Can you work these out from the model? Positions are in its coordinate system, mm. A direction names the side the tool comes from. Coordinates: 2 decimals unless noted, no trailing zeros. Write each loop counter-clockwise with the first axis right and the second up, starting at its lowest first coordinate (ties: lowest second). Pieces come first, ordered by that corner, then holes. Notation, with made-up numbers: (-6, -16) -> (1, -16) arc R15 ccw to (1, 10) -> close; hole circle Ø8 at (47.25, 84.5). An arc over 180 degrees is marked (long way). Use one line per item in the form item = value.
```python
from build123d import *

# Parameters (mm, degrees)
SKETCH1_W           = 110.236
SKETCH1_H           = 89.916
BOSS_EXTRUDE1_DEPTH = 17.78
SKETCH2_W           = 19.05
SKETCH2_H           = 12.7
CUT_EXTRUDE1_DEPTH  = 17.78


with BuildPart() as part:
    # Sketch1 → Boss-Extrude1 (new body)
    with BuildSketch(Plane(origin=(0, 0, 0), x_dir=(1, 0, 0), z_dir=(0, 1, 0))):
        with Locations((0, -19.671907216)):
            Rectangle(SKETCH1_W, SKETCH1_H)
    extrude(amount=BOSS_EXTRUDE1_DEPTH)

    # Sketch2 → Cut-Extrude1 (cut)
    with BuildSketch(Plane(origin=(0, 17.78, 0), x_dir=(1, 0, 0), z_dir=(0, 1, 0))):
        with Locations((-45.593, -58.279907216)):
            Rectangle(SKETCH2_W, SKETCH2_H)
        with Locations((45.593, -58.279907216)):
            Rectangle(SKETCH2_W, SKETCH2_H)
    extrude(amount=-CUT_EXTRUDE1_DEPTH, mode=Mode.SUBTRACT)


solid = part.part
```
Q1. Suppose I cut it at A-A (y = 6.75). Write out the boundary of the cut face in (x, z).
Return value:
outline = (-55.12, -25.29) -> (55.12, -25.29) -> (55.12, 51.93) -> (36.07, 51.93) -> (36.07, 64.63) -> (-36.07, 64.63) -> (-36.07, 51.93) -> (-55.12, 51.93) -> close
Q2. If I drill on line 1 (Z direction, x = -40, y = 8.5); line 2 (X direction, y = 13.75, z = 58.5), over which ranges is the centre line in solid material (lowest first)? Write a range as from..to.
Return value:
line_1 = -25.29..51.93
line_2 = -36.07..36.07
Q3. Will these pins go through, and if not, where does the flat tip stop? pin 1 (5.5 mm diameter, centred on x = -45, y = 12.5, fed in from +Z); pin 2 (4 mm diameter, centred on y = 14.5, z = 55.5, fed in from -X); pin 3 (10 mm diameter, centred on y = 7.5, z = 59.5, fed in from +X).
Return value:
pin_1 = 51.93
pin_2 = -36.07
pin_3 = 36.07
Q4. Suppose I cut it at B-B (x = -38.5). Write out the boundary of the cut face in (y, z), then the cut area to 3 significant figures.
Return value:
outline = (0, -25.29) -> (17.78, -25.29) -> (17.78, 51.93) -> (0, 51.93) -> close
area = 1,370 mm2
Q5. For faces 1 (the flat face through (-55.118, 9, 14)), 2 (the flat face through (-46, 9, 51.93)), 3 (the flat face through (45, 9, 51.93)), which set-ups out of +Z, -Z, +X, -X, +Y, -Y let a thin tool reach every point of the face, with its end or its side?
Return value:
face_1 = +Z, -Z, -X, +Y, -Y
face_2 = +Z, -X, +Y, -Y
face_3 = +Z, +X, +Y, -Y
